The model under review builds one solid part; all positions refer to its coordinate system, in mm. A direction names the side the tool comes from. Round coordinates to 2 decimals unless told otherwise and drop trailing zeros. Loops run counter-clockwise (first coordinate to the right, second up) from the corner with the lowest first, then second, coordinate; pieces in that order, holes last. Notation, with made-up numbers: (4, 82) -> (16, 82) arc R31 cw to (16, 111) -> close; hole circle Ø6 at (-29, 67). An arc over 180 degrees is marked (long way). Use a Markdown table: item, result. Add a question column.
1) Mouldability with a two-part tool opening along Y and no side actions: class faces 6 (the flat face through (2, 8, 0)), 7 (the flat face through (-2, 55, 0)), 8 (the flat face through (2, 17, 0)), 9 (the flat face through (-3.5, 27, 0)) as released by +Y, released by -Y, zero draft, split by the parting line, or undercut.
2) Insertion check: pin 1 (0.8 mm diameter, centred on x = 0, z = 0.5, fed in from +Y); pin 2 (1.2 mm diameter, centred on x = -0.5, z = 0, fed in from -Y); pin 3 (2 mm diameter, centred on y = 14, z = -0.5, fed in from +X). Each pin has a flat end and moves straight along its axis. Give the tip position at first contact, or say it passes through.
3) Consider section C-C on x = 0. Give the boundary of the cut face in (y, z), plus the area to 4 significant figures.
4) Consider section D-D on y = 15.5. Give the boundary of the cut face in (x, z), plus the area to 3 significant figures.
5) Wall thickness on probe 1 along X at (y, z) = (1.9, 0); probe 2 along Y at (x, z) = (0.75, -0.25); probe 3 along Y at (x, z) = (2.5, -1): over which ranges is each line inside the solid? List them lowest first.
6) For faces 1 (the flat face through (-2, 0, 0)), 2 (the cylindrical face through (1.22, 2.54, -0.27)), 3 (the flat face through (0, 27, -3.5)), 4 (the flat face through (0, 43, 0)), 5 (the flat face through (0.5, 13, 0)), list the 3-axis set-ups (+Z, -Z, +X, -X, +Y, -Y) from which the entire face can be reached by the end or side of a thin tool; tool diameter is ignored.
7) Consider section B-B on z = 2.75. Give the boundary of the cut face in (x, y), plus the area to 3 significant figures.
8) Consider section A-A on x = 2.5. Give the boundary of the cut face in (y, z).
from build123d import *

# Parameters (mm, degrees)
BOSS_EXTRUDE1_DEPTH = 55
SKETCH2_R           = 1.25
CUT_EXTRUDE1_DEPTH  = 12
SKETCH4_W           = 7
SKETCH4_H           = 9
CUT_EXTRUDE3_DEPTH  = 3
CUT_EXTRUDE4_START  = -5
SKETCH3_R           = 1.25
CUT_EXTRUDE4_DEPTH  = 5


with BuildPart() as part:
    # Sketch1 → Boss-Extrude1 (new body)
    with BuildSketch(Plane(origin=(0, 0, 0), x_dir=(1, 0, 0), z_dir=(0, 1, 0))):
        Polygon((0, 3.5), (-3.5, 3.5), (-3.5, -3.5), (3.5, -3.5), (3.5, 3.5), align=None)
    extrude(amount=BOSS_EXTRUDE1_DEPTH)

    # Sketch2 → Cut-Extrude1 (cut)
    with BuildSketch(Plane(origin=(0, 55, 0), x_dir=(1, 0, 0), z_dir=(0, 1, 0))):
        with Locations(Location((0, 0, 0), (0, 0, 270))):
            Circle(SKETCH2_R)
    extrude(amount=-CUT_EXTRUDE1_DEPTH, mode=Mode.SUBTRACT)

    # Sketch4 → Cut-Extrude3 (cut)
    with BuildSketch(Plane(origin=(3.5, 0, 0), x_dir=(0, 0, -1), z_dir=(1, 0, 0))):
        with Locations((0, 12.5)):
            Rectangle(SKETCH4_W, SKETCH4_H)
    extrude(amount=-CUT_EXTRUDE3_DEPTH, mode=Mode.SUBTRACT)

    # Sketch3 → Cut-Extrude4 (cut)
    with BuildSketch(Plane.XZ.offset(CUT_EXTRUDE4_START)):
        with Locations(Location((0, 0, 0), (0, 0, 90))):
            Circle(SKETCH3_R)
    extrude(amount=CUT_EXTRUDE4_DEPTH, mode=Mode.SUBTRACT)


solid = part.part
Result set:
| question | item | result |
|---|---|---|
| 1 | face 6 | undercut |
| 1 | face 7 | released by +Y |
| 1 | face 8 | undercut |
| 1 | face 9 | zero draft |
| 2 | pin 1 | y = 43 |
| 2 | pin 2 | y = 5 |
| 2 | pin 3 | x = 0.5 |
| 3 | outline | (0, -3.5) -> (55, -3.5) -> (55, -1.25) -> (43, -1.25) -> (43, 1.25) -> (55, 1.25) -> (55, 3.5) -> (0, 3.5) -> (0, 1.25) -> (5, 1.25) -> (5, -1.25) -> (0, -1.25) -> close |
| 3 | area | 342.5 mm2 |
| 4 | outline | (-3.5, -3.5) -> (0.5, -3.5) -> (0.5, 3.5) -> (-3.5, 3.5) -> close |
| 4 | area | 28.0 mm2 |
| 5 | probe 1 | -3.5 to -1.25, 1.25 to 3.5 |
| 5 | probe 2 | 5 to 8, 17 to 43 |
| 5 | probe 3 | 0 to 8, 17 to 55 |
| 6 | face 1 | +Z, -Z, +X, -X, -Y |
| 6 | face 2 | -Y |
| 6 | face 3 | -Z, +X, -X, +Y, -Y |
| 6 | face 4 | +Y |
| 6 | face 5 | +Z, -Z, +X |
| 7 | outline | (-3.5, 0) -> (3.5, 0) -> (3.5, 8) -> (0.5, 8) -> (0.5, 17) -> (3.5, 17) -> (3.5, 55) -> (-3.5, 55) -> close |
| 7 | area | 358 mm2 |
| 8 | outline | (0, -3.5) -> (8, -3.5) -> (8, 3.5) -> (0, 3.5) -> close; (17, -3.5) -> (55, -3.5) -> (55, 3.5) -> (17, 3.5) -> close |
